Source: CAD feature listing. Evaluate the final solid. Frame: model axes, mm. Round coordinates to 2 decimals unless told otherwise and drop trailing zeros. Order: outer loops, then holes, each group sorted by start corner. A loop starts at its lowest first (then second) coordinate and runs counter-clockwise, first axis right, second up. Notation, with made-up numbers: M -8.5,77 L 31.5,77 A24 ccw 31.5,97 Z; hole C 73,43.25 d2. An arc over 180 degrees is marked long. Use one line per item in the form item = value. Start each with the question number.
Q1. Section C-C (y = -8). Return the cut outline in (x, z).
Q2. Section B-B (x = -11.5). Return the cut outline in (y, z).
Q3. Contact query for flat-ended pins moving along their axis: pin 1 (3 mm diameter, centred on y = -9, z = -9, fed in from +X); pin 2 (6.5 mm diameter, centred on y = -10.5, z = -8, fed in from -X); pin 3 (6.5 mm diameter, centred on x = 86, y = -9.5, fed in from +Z). Output: stop coordinate, or through.
Q4. Section A-A (z = -8). Return the cut outline in (x, y).
Q5. Material intervals for probe 1 along Z at (x, y) = (142, -8.75); probe 2 along X at (y, z) = (-6.75, 1.5), sorted ascending.
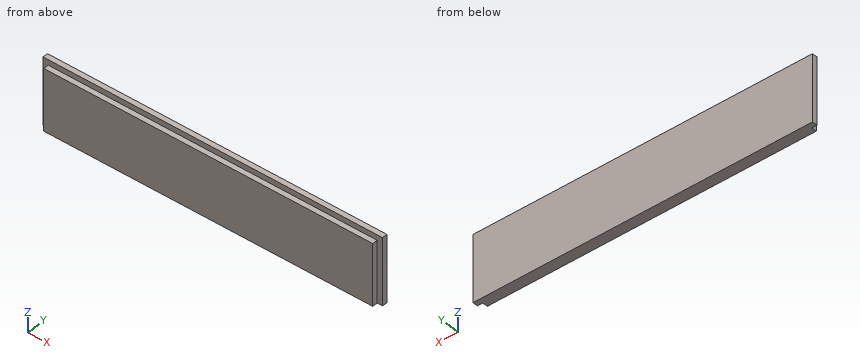
from build123d import *

# Parameters (mm, degrees)
F0_W     = 388
F0_H     = 75
F1_DEPTH = 12
F2_W     = 6
F2_H     = 75
F3_DEPTH = 6
F4_W     = 6
F4_H     = 75
F5_DEPTH = 6
F6_W     = 376
F6_H     = 6
F7_DEPTH = 6


with BuildPart() as f1:
    # F0 (on Front) → F1 (new body)
    with BuildSketch(Plane.XZ):
        with Locations((10.992817, 0)):
            Rectangle(F0_W, F0_H)
    extrude(amount=F1_DEPTH)

    # F2 (on face) → F3 (cut)
    with BuildSketch(Plane.XZ.offset(12)):
        with Locations((-180.007183, 0)):
            Rectangle(F2_W, F2_H)
    extrude(amount=-F3_DEPTH, mode=Mode.SUBTRACT)

    # F4 (on face) → F5 (cut)
    with BuildSketch(Plane.XZ.offset(12)):
        with Locations((201.992817, 0)):
            Rectangle(F4_W, F4_H)
    extrude(amount=-F5_DEPTH, mode=Mode.SUBTRACT)

    # F6 (on face) → F7 (cut)
    with BuildSketch(Plane.XZ.offset(12)):
        with Locations((10.992817, 34.5)):
            Rectangle(F6_W, F6_H)
    extrude(amount=-F7_DEPTH, mode=Mode.SUBTRACT)


solid = f1.part
Results list:
q1.outline = M -177.01,-37.5 L 198.99,-37.5 L 198.99,31.5 L -177.01,31.5 Z
q2.outline = M -12,-37.5 L 0,-37.5 L 0,37.5 L -6,37.5 L -6,31.5 L -12,31.5 Z
q3.pin_1 = 198.99
q3.pin_2 = -177.01
q3.pin_3 = 31.5
q4.outline = M -183.01,-6 L -177.01,-6 L -177.01,-12 L 198.99,-12 L 198.99,-6 L 204.99,-6 L 204.99,0 L -183.01,0 Z
q5.probe_1 = -37.5 to 31.5
q5.probe_2 = -177.01 to 198.99
